Design review of the part built by this model. Coordinates are the model's own, in mm. Face numbers are marked on the shaded views. Round coordinates to 2 decimals unless told otherwise and drop trailing zeros. Use a Markdown table: item, result.
from build123d import *

# Parameters (mm, degrees)
POST_HOLE_R             = 10
CUT_EXTRUDE1_DEPTH      = 100
CUT_EXTRUDE2_DEPTH      = 244.732583295
CUT_EXTRUDE2_DEPTH_BACK = 244.732583295


with BuildPart() as part:
    # Loft1: read off the stored shape, not the designer's step
    # Loft1: loft between two sections, ruled curve by curve
    loft1_from = [
        Edge.make_bspline([(0, 0, -65), (1.090128751, 0, -61.366237497), (3.270747147, 0, -54.097509509), (6.471517091, 0, -43.428276362), (9.544840896, 0, -33.183863681), (11.485081194, 0, -26.716396019), (12.666432162, 0, -22.77855946), (12.968402106, 0, -21.305053815), (13.100609282, 0, -19.286967133), (12.978325762, 0, -17.392629287), (12.635490493, 0, -15.578921438), (12.073950502, 0, -13.82193497), (11.281547245, 0, -12.101334039), (10.209994947, 0, -10.396029742), (9.25103095, 0, -9.25103095), (8.163446408, 0, -8.163446408), (7.044301694, 0, -7.044301694), (4.665334779, 0, -4.665334779), (1.934160234, 0, -1.934160234), (0.587535045, 0, -0.587535045), (0, 0, 0)], [0, 0, 0, 0, 0.144398069, 0.288796138, 0.433194208, 0.577592277, 0.577592277, 0.614580384, 0.651568491, 0.688556598, 0.725544706, 0.762532813, 0.79952092, 0.836509027, 0.873497134, 0.873497134, 0.905122851, 0.936748567, 0.968374284, 1, 1, 1, 1], 3),
        Edge.make_line((0, 0, -65), (0, 0, 0)),
    ]
    loft1_to = [
        Edge.make_bspline([(0, -300, -40), (0.497105388, -300, -38.202262552), (1.498303235, -300, -34.581519535), (3.037083349, -300, -29.016658037), (4.633229436, -300, -23.244337598), (5.753794564, -300, -19.191913419), (6.484300851, -300, -16.550102367), (6.736474062, -300, -15.404380913), (6.917285676, -300, -13.486434812), (6.834511282, -300, -11.412388499), (6.44022099, -300, -9.278535319), (5.736721859, -300, -7.220345405), (4.785310579, -300, -5.360639369), (3.675318905, -300, -3.765229265), (2.883667943, -300, -2.883667943), (2.143164712, -300, -2.143164712), (1.762545696, -300, -1.762545696), (1.206796855, -300, -1.206796855), (0.680514831, -300, -0.680514831), (0.288861433, -300, -0.288861433), (0, -300, 0)], [0, 0, 0, 0, 0.144398069, 0.288796138, 0.433194208, 0.577592277, 0.577592277, 0.614580384, 0.651568491, 0.688556598, 0.725544706, 0.762532813, 0.79952092, 0.836509027, 0.873497134, 0.873497134, 0.905122851, 0.936748567, 0.968374284, 1, 1, 1, 1], 3),
        Edge.make_line((0, -300, -40), (0, -300, 0)),
    ]
    loft1 = Solid(Shell([*[Face.make_surface_from_curves(loft1_from[k], loft1_to[k]) for k in range(2)], Face(Wire(loft1_from)), Face(Wire(loft1_to))]))
    add(loft1)

    # Mirror1: Loft1 across plane
    add(loft1.mirror(Plane.ZY))

    # post_hole → Cut-Extrude1 (cut)
    with BuildSketch(Plane(origin=(0, 0, 0), x_dir=(1, 0, 0), z_dir=(0, 1, 0))):
        with Locations(Location((0, 18, 0), (0, 0, 270))):
            Circle(POST_HOLE_R)
    extrude(amount=-CUT_EXTRUDE1_DEPTH, mode=Mode.SUBTRACT)

    # Sketch1 → Cut-Extrude2 (cut, two sides: drawn at the far end of the back side and taken through both)
    with BuildSketch(Plane(origin=(-1.395234412, -236.356805311, -57.724602067), x_dir=(0.03510103444042518, 0, 0.9993837688201725), z_dir=(-0.9993837688201725, 0, 0.03510103444042518)).offset(-CUT_EXTRUDE2_DEPTH_BACK)):
        with BuildLine():
            Line((-6.901046872, 232.503708167), (-7.221940435, 236.356805311))
            Line((-7.221940435, 236.356805311), (34.607125692, 236.356805311))
            Line((34.607125692, 236.356805311), (49.382745775, 236.356805311))
            Line((49.382745775, 236.356805311), (57.738004539, 236.356805311))
            Line((57.738004539, 236.356805311), (57.738004539, 220.068385372))
            add(Edge.make_bspline(
                [(-6.901046872, 232.503708167), (14.59060476, 228.075000406), (36.140920736, 223.929205599), (57.738004539, 220.068385372)],
                knots=[0.014685246, 0.014685246, 0.014685246, 0.014685246, 0.066243156, 0.066243156, 0.066243156, 0.066243156], degree=3))
        make_face()
    extrude(amount=CUT_EXTRUDE2_DEPTH + CUT_EXTRUDE2_DEPTH_BACK, mode=Mode.SUBTRACT)


solid = part.part
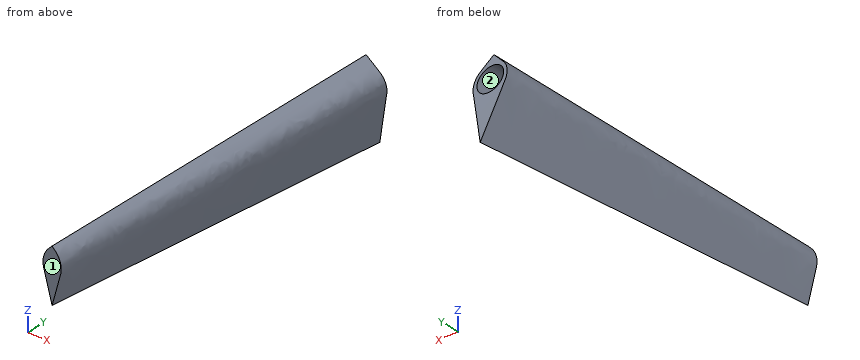
1. Insertion check: pin 1 (1.5 mm diameter, centred on y = -256, z = -35, fed in from -X); pin 2 (6 mm diameter, centred on y = -182, z = -38, fed in from -X); pin 3 (4 mm diameter, centred on x = 7, y = -189.5, fed in from +Z). Each pin has a flat end and moves straight along its axis. Give the tip position at first contact, or say it passes through.
Check values:
| item | result |
|---|---|
| pin 1 | stops at x = -2.66 |
| pin 2 | stops at x = -4.3 |
| pin 3 | stops at z = -5.01 |
2. Wall thickness on line 1 along X through (y, z) = (-51, -18); line 2 along X through (y, z) = (-69, -18); line 3 along Y through (x, z) = (-3.75, -25): over which ranges is each line inside the solid? List them lowest first. Write a range as from..to.
Check values:
| item | result |
|---|---|
| line 1 | x = -12.01..-10, 10..12.01 |
| line 2 | x = -11.64..-10, 10..11.64 |
| line 3 | y = -300..-100 |
3. The part is to be moulded in two halves that separate along Z. For the marked faces 1 and 2, say which applies: pulls with the +Z half, pulls with the -Z half, needs draft (parallel to the pull), parting line crosses it, or undercut.
Check values:
| item | result |
|---|---|
| face 1 | needs draft |
| face 2 | undercut |
